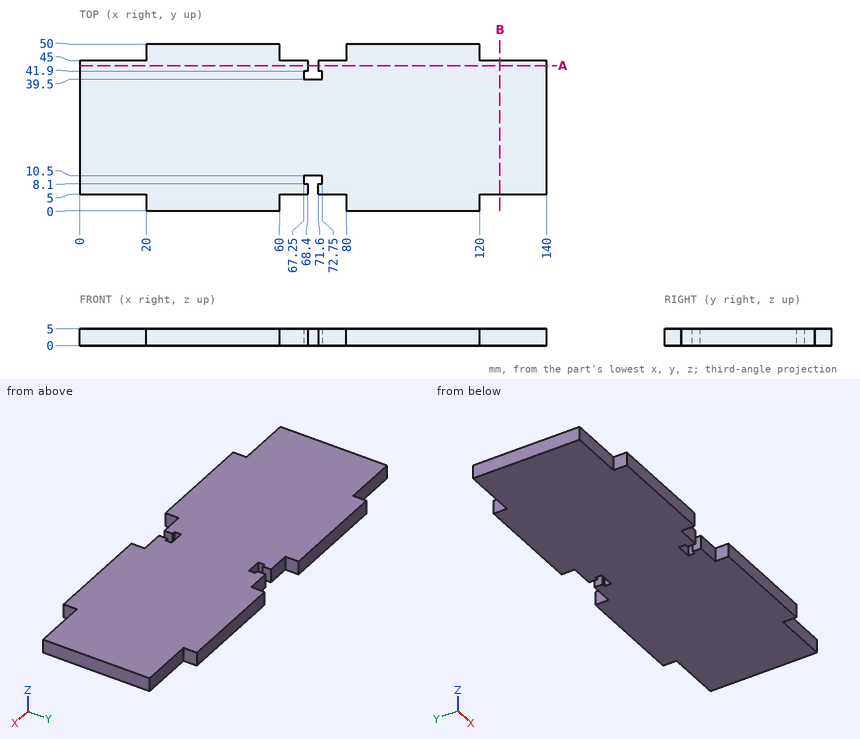
Verification items for this drawing (mm, ordinates from the low corner). Give positions to 0.01 mm unless a question says otherwise; leave off trailing zeros. Order: outer loops, then holes, each group sorted by start corner. A loop starts at its lowest first (then second) coordinate and runs counter-clockwise, first axis right, second up.
1) Material ranges on probe 1 along Y at (x, z) = (68, 3.5); probe 2 along X at (y, z) = (40, 3.5); probe 3 along Y at (x, z) = (124, 0.6), recorded low to high.
Results are:
probe 1: y = 5 to 8.1, 10.5 to 39.5, 41.9 to 45
probe 2: x = 0 to 67.25, 72.75 to 140
probe 3: y = 5 to 45
2) Cross-section at A-A (y = 43.5). Record the boundary of the cut face in (x, z), then the cut area to 3 significant figures.
Results are:
outline: (0, 0) - (68.4, 0) - (68.4, 5) - (0, 5) - close; (71.6, 0) - (140, 0) - (140, 5) - (71.6, 5) - close
area: 684 mm2
3) Gauge pin test, flat ends, axial feed: pin 1 (1.5 mm diameter, centred on y = 6, z = 3, fed in from -X); pin 2 (1.5 mm diameter, centred on x = 63, z = 3.5, fed in from -Y); pin 3 (0.6 mm diameter, centred on x = 67.5, z = 2.5, fed in from +Y); pin 4 (2.5 mm diameter, centred on y = 3, z = 3, fed in from -X). Record the tip position at first contact, or that the pin passes through.
Results are:
pin 1: stops at x = 0
pin 2: stops at y = 5
pin 3: stops at y = 45
pin 4: stops at x = 20
4) Cross-section at B-B (x = 126). Record the boundary of the cut face in (y, z), then the cut area to 3 significant figures.
Results are:
outline: (5, 0) - (45, 0) - (45, 5) - (5, 5) - close
area: 200 mm2
